```python
from build123d import *

# Parameters (mm, degrees)
SKETCH1_W           = 280
SKETCH1_H           = 120
SKETCH1_R           = 4.25
BOSS_EXTRUDE1_DEPTH = 15
SKETCH2_R           = 6.75
CUT_EXTRUDE1_DEPTH  = 10
CHAMFER2_SIZE       = 3
CHAMFER3_SIZE       = 3


with BuildPart() as part:
    # Sketch1 → Boss-Extrude1 (new body)
    with BuildSketch(Plane.XY):
        Rectangle(SKETCH1_W, SKETCH1_H)
        with Locations((-125, 45)):
            Circle(SKETCH1_R, mode=Mode.SUBTRACT)
        with Locations((125, 45)):
            Circle(SKETCH1_R, mode=Mode.SUBTRACT)
        with Locations((125, -45)):
            Circle(SKETCH1_R, mode=Mode.SUBTRACT)
        with Locations((-125, -45)):
            Circle(SKETCH1_R, mode=Mode.SUBTRACT)
    extrude(amount=BOSS_EXTRUDE1_DEPTH)

    # Sketch2 → Cut-Extrude1 (cut)
    with BuildSketch(Plane.XY.offset(15)):
        with Locations((-125, 45)):
            Circle(SKETCH2_R)
        with Locations((125, 45)):
            Circle(SKETCH2_R)
        with Locations((125, -45)):
            Circle(SKETCH2_R)
        with Locations((-125, -45)):
            Circle(SKETCH2_R)
    extrude(amount=-CUT_EXTRUDE1_DEPTH, mode=Mode.SUBTRACT)

    # Chamfer2
    # the kernel refuses this chamfer: 3 mm, written as the material it takes off along each edge
    with BuildSketch(Plane(origin=(-125, 45, 5), x_dir=(1, 0, 0), z_dir=(0, 1, 0))) as chamfer2_piece_1_section:
        Polygon((4.25, CHAMFER2_SIZE), (4.25 + CHAMFER2_SIZE, 0), (4.25, 0), align=None)
    chamfer2_piece_1 = revolve(axis=Axis((-125, 45, 5), (0, 0, -1)), mode=Mode.PRIVATE)
    chamfer2_piece_1 = chamfer2_piece_1 & Plane(origin=(-125, 45, 3.245521929), x_dir=(1, 0, 0), z_dir=(0, 0, 1)) * Cylinder(6.75, 29, mode=Mode.PRIVATE)
    add(chamfer2_piece_1, mode=Mode.SUBTRACT)

    # Chamfer3
    # the kernel refuses this chamfer: 3 mm, written as the material it takes off along each edge
    with BuildSketch(Plane(origin=(125, 45, 5), x_dir=(1, 0, 0), z_dir=(0, 1, 0))) as chamfer3_piece_1_section:
        Polygon((4.25 + CHAMFER3_SIZE, 0), (4.25, CHAMFER3_SIZE), (4.25, 0), align=None)
    chamfer3_piece_1 = revolve(axis=Axis((125, 45, 5), (0, 0, -1)), mode=Mode.PRIVATE)
    chamfer3_piece_1 = chamfer3_piece_1 & Plane(origin=(125, 45, 3.245521929), x_dir=(1, 0, 0), z_dir=(0, 0, 1)) * Cylinder(6.75, 29, mode=Mode.PRIVATE)
    add(chamfer3_piece_1, mode=Mode.SUBTRACT)
    with BuildSketch(Plane(origin=(125, -45, 5), x_dir=(1, 0, 0), z_dir=(0, 1, 0))) as chamfer3_piece_2_section:
        Polygon((4.25 + CHAMFER3_SIZE, 0), (4.25, CHAMFER3_SIZE), (4.25, 0), align=None)
    chamfer3_piece_2 = revolve(axis=Axis((125, -45, 5), (0, 0, -1)), mode=Mode.PRIVATE)
    chamfer3_piece_2 = chamfer3_piece_2 & Plane(origin=(125, -45, 3.245521929), x_dir=(1, 0, 0), z_dir=(0, 0, 1)) * Cylinder(6.75, 29, mode=Mode.PRIVATE)
    add(chamfer3_piece_2, mode=Mode.SUBTRACT)
    with BuildSketch(Plane(origin=(-125, -45, 5), x_dir=(1, 0, 0), z_dir=(0, 1, 0))) as chamfer3_piece_3_section:
        Polygon((4.25 + CHAMFER3_SIZE, 0), (4.25, CHAMFER3_SIZE), (4.25, 0), align=None)
    chamfer3_piece_3 = revolve(axis=Axis((-125, -45, 5), (0, 0, -1)), mode=Mode.PRIVATE)
    chamfer3_piece_3 = chamfer3_piece_3 & Plane(origin=(-125, -45, 3.245521929), x_dir=(1, 0, 0), z_dir=(0, 0, 1)) * Cylinder(6.75, 29, mode=Mode.PRIVATE)
    add(chamfer3_piece_3, mode=Mode.SUBTRACT)


solid = part.part
```
Input: part model. Units: mm. Frame: model coordinates. A direction names the side the tool comes from. Coordinates: 2 decimals unless noted, no trailing zeros. Write each loop counter-clockwise with the first axis right and the second up, starting at its lowest first coordinate (ties: lowest second). Pieces come first, ordered by that corner, then holes.
1) Pin query (flat end, axial travel): pin 1 Ø7.5 at (x, y) = (125, -45) entering from +Z; pin 2 Ø12 at (x, y) = (-125, 45) entering from +Z. Return the tip coordinate at first contact, or that it passes through.
2) Section B-B on y = 45. Output: boundary loops of the cut face in (x, z).
3) Section A-A on x = -125. Output: boundary loops of the cut face in (y, z).
4) Material intervals for line 1 along X through (y, z) = (-45, 1.4); line 2 along Y through (x, z) = (125, 1.5); line 3 along Y through (x, z) = (125, 10), sorted ascending.
5) Set-up query: faces 4 (the cylindrical face through (-118.765, -47.585, 9.823)), 5 (the flat face through (-140, -1, 7)). Return all of +Z, -Z, +X, -X, +Y, -Y with unobstructed straight access to the full face (end or side cutting, diameter ignored); none if empty.
6) Section C-C on z = 10.5. Output: boundary loops of the cut face in (x, y), and give its area (3 significant figures).
7) Mould query, pull axis Y, two halves, no side actions, for faces 1 (the flat face through (140, -1, 7)), 2 (the conical face through (-128.25, 42.02, 2.16)), 3 (the flat face through (-2, -60, 7)). Classes: pulls with the +Y half, pulls with the -Y half, needs draft (parallel to the pull), parting line crosses it, or undercut.
Check result:
1. pin 1: passes through
1. pin 2: stops at z = 3.75
2. outline: (-140, 0) - (-129.25, 0) - (-129.25, 2) - (-131.75, 4.5) - (-131.75, 15) - (-140, 15) - close; (-120.75, 0) - (120.75, 0) - (120.75, 2) - (118.25, 4.5) - (118.25, 15) - (-118.25, 15) - (-118.25, 4.5) - (-120.75, 2) - close; (129.25, 0) - (140, 0) - (140, 15) - (131.75, 15) - (131.75, 4.5) - (129.25, 2) - close
3. outline: (-60, 0) - (-49.25, 0) - (-49.25, 2) - (-51.75, 4.5) - (-51.75, 15) - (-60, 15) - close; (-40.75, 0) - (40.75, 0) - (40.75, 2) - (38.25, 4.5) - (38.25, 15) - (-38.25, 15) - (-38.25, 4.5) - (-40.75, 2) - close; (49.25, 0) - (60, 0) - (60, 15) - (51.75, 15) - (51.75, 4.5) - (49.25, 2) - close
4. line 1: x = -140 to -129.25, -120.75 to 120.75, 129.25 to 140
4. line 2: y = -60 to -49.25, -40.75 to 40.75, 49.25 to 60
4. line 3: y = -60 to -51.75, -38.25 to 38.25, 51.75 to 60
5. face 4: +Z
5. face 5: +Z, -Z, -X, +Y, -Y
6. outline: (-140, -60) - (140, -60) - (140, 60) - (-140, 60) - close; hole circle Ø13.5 at (-125, -45); hole circle Ø13.5 at (-125, 45); hole circle Ø13.5 at (125, -45); hole circle Ø13.5 at (125, 45)
6. area: 33,000 mm2
7. face 1: needs draft
7. face 2: undercut
7. face 3: pulls with the -Y half
